Can you work these out from the model? Positions are in its coordinate system, mm. A direction names the side the tool comes from. Give positions to 0.01 mm unless a question says otherwise; leave off trailing zeros. Loops run counter-clockwise (first coordinate to the right, second up) from the corner with the lowest first, then second, coordinate; pieces in that order, holes last. Notation, with made-up numbers: (16.5, 43) -> (54.5, 43) arc R12 cw to (54.5, 66) -> close; hole circle Ø6 at (65, 39). An arc over 180 degrees is marked (long way). Return JSON: item names as keys, results as strings. Group by question number.
Q1. Suppose I cut it at A-A, the plane y = 0. Please give me the cut outline in (x, z).
Q2. Which directions (+Z, -Z, +X, -X, +Y, -Y) give clear straight access to the entire face, cutting with the end or side of a thin tool? Please do faces 1 (the cylindrical face through (3.94, 8.93, -11.64)), 2 (the flat face through (21.933, 4, -13)), 3 (the flat face through (27, -3, 5)), 4 (the flat face through (8, -9, 10)), 5 (the flat face through (0, 6, 0)).
Q3. Thinking about a two-plate mould opening in Z: for faces 6 (the cylindrical face through (13.69, 5.37, -1.19)), 7 (the cylindrical face through (13.43, -0.88, -19.98)), 8 (the flat face through (12.933, 4, 13)), which applies, pulls with the +Z half, pulls with the -Z half, needs draft (parallel to the pull), parting line crosses it, or undercut?
Q4. I need wall thicknesses on line 1 along Y through (x, z) = (10, 0); line 2 along X through (y, z) = (19, 3); line 3 along Z through (x, y) = (2.25, 4). Which ranges of each line are inside material? Lowest first, please. Write a range as [from, to].
Q5. Suppose I cut it at B-B, the plane x = 6.5. Please give me the cut outline in (y, z), and give its area (3 significant figures).
Q6. Will these pins go through, and if not, where does the flat tip stop? pin 1 (12 mm diameter, centred on x = 4, z = 12, fed in from -Y); pin 2 (12 mm diameter, centred on x = 3, y = -10.5, fed in from -Z); pin 3 (2 mm diameter, centred on x = 12, z = -4, fed in from +Y).
```python
from build123d import *

# Parameters (mm, degrees)
F_3_5_3_5_DIAMETER_HOLE1_D     = 3.5
F_3_5_3_5_DIAMETER_HOLE1_DEPTH = 12
F_3_5_3_5_DIAMETER_HOLE1_TIP   = 1.75


with BuildPart() as part:
    # Sketch2 → Revolve1 (revolve)
    with BuildSketch(Plane.XY, mode=Mode.PRIVATE) as revolve1_sk:
        with BuildLine():
            Line((0, 5.5), (27, 5.5))
            Line((27, 5.5), (27, 11))
            ThreePointArc((27, 11), (24.244097244, 11.565328291), (21.93333443, 13.17))
            Line((21.93333443, 13.17), (21.93333443, 20))
            ThreePointArc((21.93333443, 20), (17.93333443, 24), (13.93333443, 20))
            Line((13.93333443, 20), (12.93333443, 20))
            Line((12.93333443, 20), (12.93333443, 13.17))
            Line((12.93333443, 13.17), (8, 13.17))
            Line((8, 13.17), (8, 14.67))
            Line((8, 14.67), (0, 14.67))
            Line((0, 14.67), (0, 5.5))
        make_face()
    revolve(revolve1_sk.sketch.rotate(Axis((0, 0, 0), (1, 0, 0)), 90), axis=Axis((0, 0, 0), (1, 0, 0)))

    # Ø3.5 (3.5) Diameter Hole1
    with Locations(Plane(origin=(23.970221342, 11.398844084, 2.591218084), x_dir=(0.897145620837, -0.441734914867, 0), z_dir=(0.432825522508, 0.879051007823, 0.19982840817))):
        with Locations((0, 0)):
            Hole(F_3_5_3_5_DIAMETER_HOLE1_D / 2, depth=F_3_5_3_5_DIAMETER_HOLE1_DEPTH)
            with Locations((0, 0, -(F_3_5_3_5_DIAMETER_HOLE1_DEPTH + F_3_5_3_5_DIAMETER_HOLE1_TIP / 2))):  # 90° drill point
                Cone(0, F_3_5_3_5_DIAMETER_HOLE1_D / 2, F_3_5_3_5_DIAMETER_HOLE1_TIP, mode=Mode.SUBTRACT)


solid = part.part
```
Ans:
{
 "1": {"outline": "(0, -14.67) -> (8, -14.67) -> (8, -13.17) -> (12.93, -13.17) -> (12.93, -20) -> (13.93, -20) arc R4 ccw to (21.93, -20) -> (21.93, -13.17) arc R7 cw to (27, -11) -> (27, -5.5) -> (0, -5.5) -> close; (0, 5.5) -> (27, 5.5) -> (27, 11) arc R7 cw to (21.93, 13.17) -> (21.93, 20) arc R4 ccw to (13.93, 20) -> (12.93, 20) -> (12.93, 13.17) -> (8, 13.17) -> (8, 14.67) -> (0, 14.67) -> close"},
 "2": {"face 1": "-X", "face 2": "+X", "face 3": "+Z, -Z, +X, +Y, -Y", "face 4": "none", "face 5": "+Z, -Z, -X, +Y, -Y"},
 "3": {"face 6": "undercut", "face 7": "parting line crosses it", "face 8": "needs draft"},
 "4": {"line 1": "y = [-13.17, -5.5], [5.5, 13.17]", "line 2": "x = [12.93, 21.93]", "line 3": "z = [-14.11, -3.77], [3.77, 14.11]"},
 "5": {"outline": "circle Ø29.34 at (0, 0); hole circle Ø11 at (0, 0)", "area": "581 mm^2"},
 "6": {"pin 1": "stops at y = -13.39", "pin 2": "stops at z = -13.96", "pin 3": "stops at y = 19.67"}
}
